Could you check a few things on this model? Use its own coordinates, in mm. Coordinates: 2 decimals unless noted, no trailing zeros. Loops run counter-clockwise (first coordinate to the right, second up) from the corner with the lowest first, then second, coordinate; pieces in that order, holes last. Notation, with made-up numbers: M -39,-13 L -35,-13 A15 cw -35,15 Z; hole C 49.25,79 d11. An arc over 180 degrees is marked long. Write each question's results on one line, items separated by ' | '.
```python
from build123d import *

# Parameters (mm, degrees)
F1_DEPTH = 2


with BuildPart() as f1:
    # F0 (on Front) → F1 (new body)
    with BuildSketch(Plane.XZ):
        with BuildLine():
            Line((7.582128, 0), (15.582128, 0))
            Line((15.582128, 0), (5.60828, 14.98407))
            ThreePointArc((5.60828, 14.98407), (0, 11.116486), (-5.60828, 14.98407))
            Line((-5.60828, 14.98407), (-11.662617, 5.888422))
            Line((-11.662617, 5.888422), (-15.582128, 0))
            Line((-15.582128, 0), (-7.582128, 0))
            Line((-7.582128, 0), (-4.5, 7.679838))
            Line((-4.5, 7.679838), (4.5, 7.679838))
            Line((4.5, 7.679838), (7.582128, 0))
        make_face()
        Polygon((-11.662617, 5.888422), (-5.60828, 14.98407), (-5.730158, 17.515007), (-8.504199, 17.560361), (-8.686104, 20.440266), (-13.597518, 20.440266), (-13.597518, 14.98407), align=None)
    extrude(amount=F1_DEPTH)


solid = f1.part
```
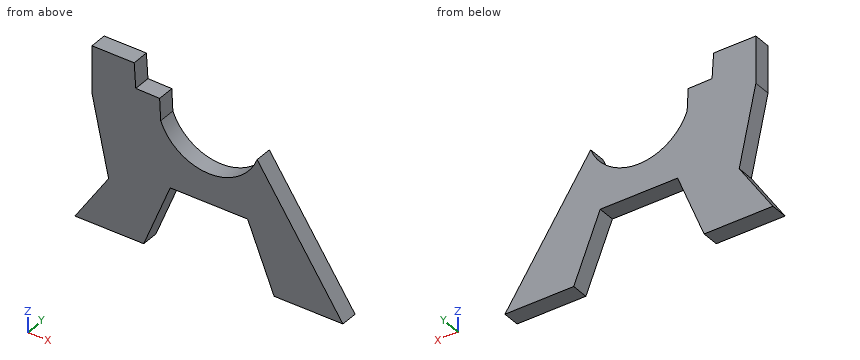
(1) Imagine slicing it at B-B, the plane x = -13. List the corners of the cut face in (y, z) for me.
Reported:
outline: M -2,0 L 0,0 L 0,3.88 L -2,3.88 Z; M -2,12.18 L 0,12.18 L 0,20.44 L -2,20.44 Z
(2) Will these pins go through, and if not, where does the flat tip stop? P1, Ø0.6, axis at x = 1.5, y = -1, coming from the -Z side; P2, Ø6, axis at x = 11.5, z = 5, coming from the +Y side.
Reported:
P1: stops at z = 7.68 | P2: stops at y = 0
(3) Imagine slicing it at A-A, the plane z = 14.25. List the corners of the cut face in (x, y) for me, and give its area (3 significant figures).
Reported:
outline: M -13.44,-2 L -5.27,-2 L -5.27,0 L -13.44,0 Z; M 5.27,-2 L 6.1,-2 L 6.1,0 L 5.27,0 Z | area: 18.0 mm2
(4) Imagine slicing it at D-D, the plane x = 0. List the corners of the cut face in (y, z) for me, and give its area (3 significant figures).
Reported:
outline: M -2,7.68 L 0,7.68 L 0,11.12 L -2,11.12 Z | area: 6.87 mm2
(5) Please list where these lines run through material, in increasing order: probe 1 along Z at (x, y) = (0, -1.8); probe 2 along X at (y, z) = (-1.05, 13.75) (3 decimals); probe 3 along Z at (x, y) = (-8, -0.3). Write a range as from..to.
Reported:
probe 1: z = 7.68..11.12 | probe 2: x = -13.335..-4.967, 4.967..6.43 | probe 3: z = 0..17.55
(6) Imagine slicing it at C-C, the plane y = -0.85. List the corners of the cut face in (x, z) for me (3 decimals), and give its area (3 significant figures).
Reported:
outline: M -15.582,0 L -7.582,0 L -4.5,7.68 L 4.5,7.68 L 7.582,0 L 15.582,0 L 5.608,14.984 A6 cw -5.608,14.984 L -5.73,17.515 L -8.504,17.56 L -8.686,20.44 L -13.598,20.44 L -13.598,14.984 L -11.663,5.888 Z | area: 264 mm2
